from build123d import *

# Parameters (mm, degrees)
SWEEP1_PROFILE_R = 2.25
CHAMFER1_SIZE    = 1
SCALE1_SCALE     = 0.8


with BuildPart() as part:
    # Sweep1: sweep along a path in Sketch1
    with BuildLine(Plane.XY) as sweep1_path:
        Line((0, 0), (16, 0))
    # Sweep1 profile (on start of the path) → Sweep1 (sweep)
    with BuildSketch(Plane(origin=(0, 0, 0), x_dir=(0, 0, 1), z_dir=(1, 0, 0))):
        Circle(SWEEP1_PROFILE_R)
    sweep(path=sweep1_path.line)

    # Chamfer1
    chamfer1_edges = [part.edges().sort_by_distance(p)[0] for p in [
        (0, 0, -2.25),
        (16, 0, -2.25),
    ]]
    chamfer(chamfer1_edges, length=CHAMFER1_SIZE)


with BuildPart() as part_1:
    # Scale1: scaled about (8, 0, 0)
    add(part.part.scale(SCALE1_SCALE).moved(Location((1.6, 0, 0))))


solid = part_1.part
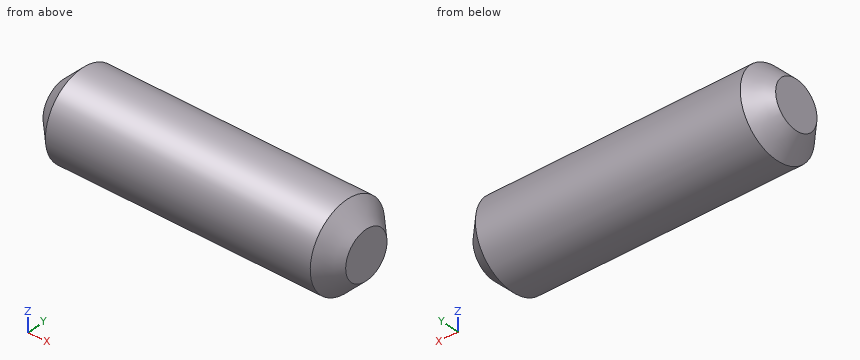
Geometry check sheet. Reference: the model listing, model coordinates, mm. Give positions to 0.01 mm unless a question says otherwise; leave off trailing zeros. Loops run counter-clockwise (first coordinate to the right, second up) from the corner with the lowest first, then second, coordinate; pieces in that order, holes last. Notation, with made-up numbers: M 24.25,-29.75 L 53.25,-29.75 A15 cw 53.25,-8.75 Z; hole C -12,82 d4. An arc over 180 degrees is marked long. Answer as a JSON object with one key per item and string values. Group by question number.
Item 1: Sectioned sample at D-D on x = 7.75. Record the boundary of the cut face in (y, z), plus the area to 3 significant figures.
Item 2: Sectioned sample at A-A on y = 0. Record the boundary of the cut face in (x, z), plus the area to 3 significant figures.
Item 3: Sectioned sample at C-C on x = 13.75. Record the boundary of the cut face in (y, z), plus the area to 3 significant figures.
Item 4: Material ranges on L1, parallel to Z at x = 4, y = -0.45; L2, parallel to Z at x = 6, y = 0.3; L3, parallel to Y at x = 7.5, z = -0.6, recorded low to high.
Findings below:
{
 "1": {"outline": "C 0,0 d3.6", "area": "10.2 mm2"},
 "2": {"outline": "M 1.6,-1 L 2.4,-1.8 L 13.6,-1.8 L 14.4,-1 L 14.4,1 L 13.6,1.8 L 2.4,1.8 L 1.6,1 Z", "area": "44.8 mm2"},
 "3": {"outline": "C 0,0 d3.3", "area": "8.55 mm2"},
 "4": {"L1": "-1.74 to 1.74", "L2": "-1.77 to 1.77", "L3": "-1.7 to 1.7"}
}
